from build123d import *

# Parameters (mm, degrees)
SKETCH_1_R      = 1.5
EXTRUDE_1_DEPTH = 56.175
EXTRUDE_START   = -9.3
SKETCH_2_R      = 2.25
EXTRUDE_2_DEPTH = 70.6
EXTRUDE_START_2 = -29.1
SKETCH_3_R      = 2.25
EXTRUDE_3_DEPTH = 19.8


with BuildPart() as part:
    # 草图1 → 凸台-拉伸1 (new, symmetric)
    with BuildSketch(Plane(origin=(0, 0, 0), x_dir=(1, 0, 0), z_dir=(0, 1, 0))):
        with Locations(Location((0, 0, 0), (0, 0, 90))):
            Circle(SKETCH_1_R)
    extrude(amount=EXTRUDE_1_DEPTH, both=True)

    # 草图2 → 凸台-拉伸2 (add)
    with BuildSketch(Plane.XZ.offset(56.175).offset(EXTRUDE_START)):
        with Locations(Location((0, 0, 0), (0, 0, 270))):
            Circle(SKETCH_2_R)
    extrude(amount=-EXTRUDE_2_DEPTH)

    # 草图3 → 凸台-拉伸3 (add)
    with BuildSketch(Plane(origin=(0, 56.175, 0), x_dir=(1, 0, 0), z_dir=(0, 1, 0)).offset(EXTRUDE_START_2)):
        with Locations(Location((0, 0, 0), (0, 0, 90))):
            Circle(SKETCH_3_R)
    extrude(amount=EXTRUDE_3_DEPTH)


solid = part.part
For this review, take the finished solid that the model builds, in its own axes (mm). A direction names the side the tool comes from. Give positions to 0.01 mm unless a question says otherwise; leave off trailing zeros. Loops run counter-clockwise (first coordinate to the right, second up) from the corner with the lowest first, then second, coordinate; pieces in that order, holes last.
Item 1: Tool access review of faces 5 (the cylindrical face through (-0.45, -51.46, -1.43)), 6 (the cylindrical face through (-0.45, 51.59, -1.43)), 7 (the flat face through (0, 23.725, 2)), 8 (the cylindrical face through (0.676, -12.069, -2.146)): name each direction out of +Z, -Z, +X, -X, +Y, -Y from which nothing blocks a thin tool from reaching the whole face with its end or side.
Item 2: Take a section at C-C, the plane y = -8. State the section outline as (x, z) points.
Item 3: Take a section at B-B, the plane z = 0. State the section outline as (x, y) points (3 decimals).
Item 4: For line 1 along Y through (x, z) = (1.9, 0.35) (3 decimals); line 2 along X through (y, z) = (46, -0.3); line 3 along X through (y, z) = (-48, 0.2), list the stretches that pass through material, from the lowest coordinate up.
Item 5: Take a section at A-A, the plane x = 0. State the section outline as (y, z) points (3 decimals).
Item 6: Draft analysis for pull direction Y (two halves, no side actions). For faces 1 (the flat face through (0, 27.075, 2)), 2 (the cylindrical face through (-0.676, 36.836, -2.146)), 3 (the flat face through (0, 46.875, 2)), 4 (the cylindrical face through (-0.45, 25.42, -1.43)), state which applies: +Y half, -Y half, draft (parallel to the pull), parting line (faces both ways), or undercut.
Item 7: Insertion check: pin 1 (1.5 mm diameter, centred on y = 19, z = 2, fed in from +X). The pin has a flat end and moves straight along its axis. Give the tip position at first contact, or say it passes through.
Calculated:
1. face 5: -Y
1. face 6: +Y
1. face 7: none
1. face 8: +Y, -Y
2. outline: circle Ø4.5 at (0, 0)
3. outline: (-2.25, -46.875) - (-1.5, -46.875) - (-1.5, -56.175) - (1.5, -56.175) - (1.5, -46.875) - (2.25, -46.875) - (2.25, 23.725) - (1.5, 23.725) - (1.5, 27.075) - (2.25, 27.075) - (2.25, 46.875) - (1.5, 46.875) - (1.5, 56.175) - (-1.5, 56.175) - (-1.5, 46.875) - (-2.25, 46.875) - (-2.25, 27.075) - (-1.5, 27.075) - (-1.5, 23.725) - (-2.25, 23.725) - close
4. line 1: y = -46.875 to 23.725, 27.075 to 46.875
4. line 2: x = -2.23 to 2.23
4. line 3: x = -1.49 to 1.49
5. outline: (-56.175, -1.5) - (-46.875, -1.5) - (-46.875, -2.25) - (23.725, -2.25) - (23.725, -1.5) - (27.075, -1.5) - (27.075, -2.25) - (46.875, -2.25) - (46.875, -1.5) - (56.175, -1.5) - (56.175, 1.5) - (46.875, 1.5) - (46.875, 2.25) - (27.075, 2.25) - (27.075, 1.5) - (23.725, 1.5) - (23.725, 2.25) - (-46.875, 2.25) - (-46.875, 1.5) - (-56.175, 1.5) - close
6. face 1: undercut
6. face 2: draft
6. face 3: +Y half
6. face 4: undercut
7. pin 1: stops at x = 1.87
